Read the model definition and answer for the solid it produces. Units are mm, in the model's axes. Face numbers are marked on the shaded views. A direction names the side the tool comes from. Coordinates: 2 decimals unless noted, no trailing zeros. Loops run counter-clockwise (first coordinate to the right, second up) from the corner with the lowest first, then second, coordinate; pieces in that order, holes last.
Q1. Section B-B (z = 1) is taken. Give the vertices of the cut face in (x, y), then the cut area to 3 significant figures.
Q2. Flat-ended cylindrical pins translate along their axes: P1, Ø2, axis at x = 16.5, z = -33.5, coming from the +Y side; P2, Ø1.8, axis at x = -22, z = 32.5, coming from the +Y side; P3, Ø0.5, axis at y = 4.5, z = -0.5, coming from the -X side. Find the tip coordinate at first contact, or state that the pin passes through.
Q3. Which of the six approach directions +Z, -Z, +X, -X, +Y, -Y give full straight-line access (tool end or side, diameter ignored) to the marked faces 1 and 2?
Q4. Section A-A (x = 3.5) is taken. Give the vertices of the cut face in (y, z), then the cut area to 3 significant figures.
Q5. Section D-D (y = 2.6) is taken. Count the separate pieces of the cut face and the enclosed holes in it, then the cut area to 3 significant figures.
Q6. Section C-C (x = -13.5) is taken. Give the vertices of the cut face in (y, z).
Q7. Straight lines are drawn through the part: line 1 (X direction, y = 1.95, z = 32.4); line 2 (X direction, y = 2.1, z = 47.9); line 3 (X direction, y = 2.1, z = 35.5). For each, find the intervals that lie inside material, in ascending order.
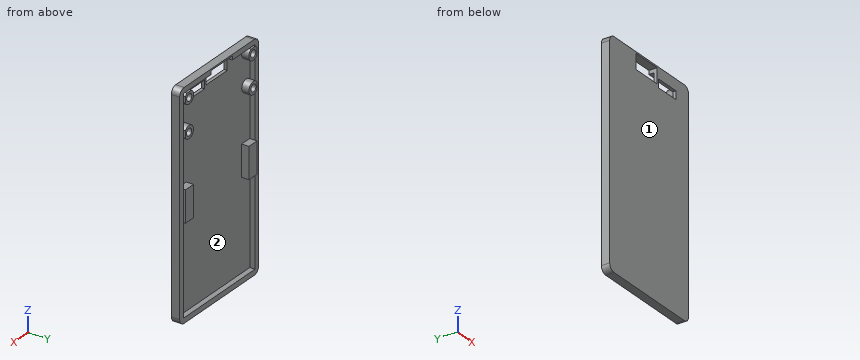
from build123d import *

# Parameters (mm, degrees)
SKETCH1_W           = 49
SKETCH1_H           = 101
BOSS_EXTRUDE1_DEPTH = 1.5
SKETCH2_W           = 54
SKETCH2_H           = 106
SKETCH2_W_2         = 49
SKETCH2_H_2         = 101
BOSS_EXTRUDE2_DEPTH = 4
SKETCH3_W           = 5.5
SKETCH3_H           = 15
BOSS_EXTRUDE3_DEPTH = 5
SKETCH4_R           = 1.75
CUT_EXTRUDE1_DEPTH  = 4.25
SKETCH5_R           = 1.75
CUT_EXTRUDE2_DEPTH  = 4.25
SKETCH6_W           = 14.5
SKETCH6_H           = 7.3
CUT_EXTRUDE3_DEPTH  = 60.690870324
SKETCH7_W           = 11.8
SKETCH7_H           = 4
CUT_EXTRUDE4_DEPTH  = 60.690870324
FILLET1_R           = 3


with BuildPart() as part:
    # Sketch1 → Boss-Extrude1 (new body)
    with BuildSketch(Plane(origin=(0, 0, 0), x_dir=(1, 0, 0), z_dir=(0, 1, 0))):
        Rectangle(SKETCH1_W, SKETCH1_H)
    extrude(amount=BOSS_EXTRUDE1_DEPTH)

    # Sketch2 → Boss-Extrude2 (add)
    with BuildSketch(Plane(origin=(0, 0, 0), x_dir=(1, 0, 0), z_dir=(0, 1, 0))):
        Rectangle(SKETCH2_W, SKETCH2_H)
        Rectangle(SKETCH2_W_2, SKETCH2_H_2, mode=Mode.SUBTRACT)
    extrude(amount=BOSS_EXTRUDE2_DEPTH)

    # Sketch3 → Boss-Extrude3 (add)
    with BuildSketch(Plane(origin=(0, 0, 0), x_dir=(1, 0, 0), z_dir=(0, 1, 0))):
        with BuildLine():
            Line((-24.5, -30.741687605), (-24.5, -34.058312395))
            ThreePointArc((-24.5, -34.058312395), (-19, -32.4), (-24.5, -30.741687605))
        make_face()
        with Locations((-21.75, 0)):
            Rectangle(SKETCH3_W, SKETCH3_H)
        with BuildLine():
            Line((-24.5, -46.403337045), (-24.5, -49.396662955))
            ThreePointArc((-24.5, -49.396662955), (-24.021320344, -50.021320344), (-23.396662955, -50.5))
            Line((-23.396662955, -50.5), (-20.403337045, -50.5))
            ThreePointArc((-20.403337045, -50.5), (-19.778679656, -45.778679656), (-24.5, -46.403337045))
        make_face()
    boss_extrude3 = extrude(amount=BOSS_EXTRUDE3_DEPTH)

    # Mirror1: Boss-Extrude3 across plane
    add(boss_extrude3.mirror(Plane(origin=(0, 0, 0), x_dir=(0, 0, 1), z_dir=(1, 0, 0))))

    # Sketch4 → Cut-Extrude1 (cut)
    with BuildSketch(Plane(origin=(0, 5, 0), x_dir=(1, 0, 0), z_dir=(0, 1, 0))):
        with Locations(Location((-21.9, -47.9, 0), (0, 0, 270))):
            Circle(SKETCH4_R)
        with Locations(Location((21.9, -47.9, 0), (0, 0, 270))):
            Circle(SKETCH4_R)
    extrude(amount=-CUT_EXTRUDE1_DEPTH, mode=Mode.SUBTRACT)

    # Sketch5 → Cut-Extrude2 (cut)
    with BuildSketch(Plane(origin=(0, 5, 0), x_dir=(1, 0, 0), z_dir=(0, 1, 0))):
        with Locations(Location((-22, -32.4, 0), (0, 0, 270))):
            Circle(SKETCH5_R)
        with Locations(Location((22, -32.4, 0), (0, 0, 270))):
            Circle(SKETCH5_R)
    extrude(amount=-CUT_EXTRUDE2_DEPTH, mode=Mode.SUBTRACT)

    # Sketch6 → Cut-Extrude3 (cut, through all)
    with BuildSketch(Plane(origin=(0, 0, 0), x_dir=(1, 0, 0), z_dir=(0, 1, 0))):
        with Locations((-1.75, -48.65)):
            Rectangle(SKETCH6_W, SKETCH6_H)
    extrude(amount=CUT_EXTRUDE3_DEPTH, mode=Mode.SUBTRACT)

    # Sketch7 → Cut-Extrude4 (cut, through all)
    with BuildSketch(Plane(origin=(0, 0, 0), x_dir=(1, 0, 0), z_dir=(0, 1, 0))):
        with Locations((12.4, -45.7)):
            Rectangle(SKETCH7_W, SKETCH7_H)
    extrude(amount=CUT_EXTRUDE4_DEPTH, mode=Mode.SUBTRACT)

    # Fillet1
    fillet1_edges = [part.edges().sort_by_distance(p)[0] for p in [
        (-27, 2, 53),
        (27, 2, 53),
        (27, 2, -53),
        (-27, 2, -53),
    ]]
    fillet(fillet1_edges, radius=FILLET1_R)


solid = part.part
Numbers:
1. outline: (-27, 0) - (27, 0) - (27, 4) - (24.5, 4) - (24.5, 5) - (19, 5) - (19, 1.5) - (-19, 1.5) - (-19, 5) - (-24.5, 5) - (-24.5, 4) - (-27, 4) - close
1. area: 132 mm2
2. P1: stops at y = 1.5
2. P2: stops at y = 0.75
2. P3: stops at x = -24.5
3. face 1: +Z, -Z, +X, -X, -Y
3. face 2: +Y
4. outline: (0, -53) - (4, -53) - (4, -50.5) - (1.5, -50.5) - (1.5, 45) - (0, 45) - close; (0, 52.3) - (4, 52.3) - (4, 53) - (0, 53) - close
4. area: 156 mm2
5. separate pieces: 1
5. enclosed holes: 7
5. area: 975 mm2
6. outline: (0, -53) - (4, -53) - (4, -50.5) - (1.5, -50.5) - (1.5, 50.5) - (4, 50.5) - (4, 53) - (0, 53) - close
7. line 1: x = -27 to -23.75, -20.25 to -19, 19 to 20.25, 23.75 to 27
7. line 2: x = -27 to -23.65, -20.15 to -18.9, 18.9 to 20.15, 23.65 to 27
7. line 3: x = -27 to -24.5, 24.5 to 27
